Drawing for the job (mm, zero at the part's lowest x, y, z). Coordinates: 2 decimals unless noted, no trailing zeros. Write each loop counter-clockwise with the first axis right and the second up, starting at its lowest first coordinate (ties: lowest second). Pieces come first, ordered by that corner, then holes. Notation, with made-up numbers: (-10.75, -23.75) -> (13.25, -23.75) arc R20 ccw to (13.25, 5.25) -> close; hole circle Ø5 at (15.5, 78.25). An arc over 180 degrees is marked (long way). Write each question's results on one line, items separated by ' | '. Start each with the question number.
Q1. Saw through at A-A on y = 50. Give the cut face in (x, z).
Q2. Saw through at D-D on x = 2.1. Count the separate pieces of the cut face and the enclosed holes in it, and give its area (3 significant figures).
Q3. Saw through at C-C on y = 32. Give the cut face in (x, z).
Q4. Drop a flat-ended pin along its axis: pin 1 Ø5 at (y, z) = (85.39, 75.72) entering from -X. Give the stop position or say it passes through.
Q5. Drill centre lines: line 1 (Y direction, x = 1.1, z = 50); line 2 (Y direction, x = 0.9, z = 91) (1 decimal); line 3 (Z direction, x = 0.4, y = 73.5) (1 decimal). Where is each one in solid material? Low to high.
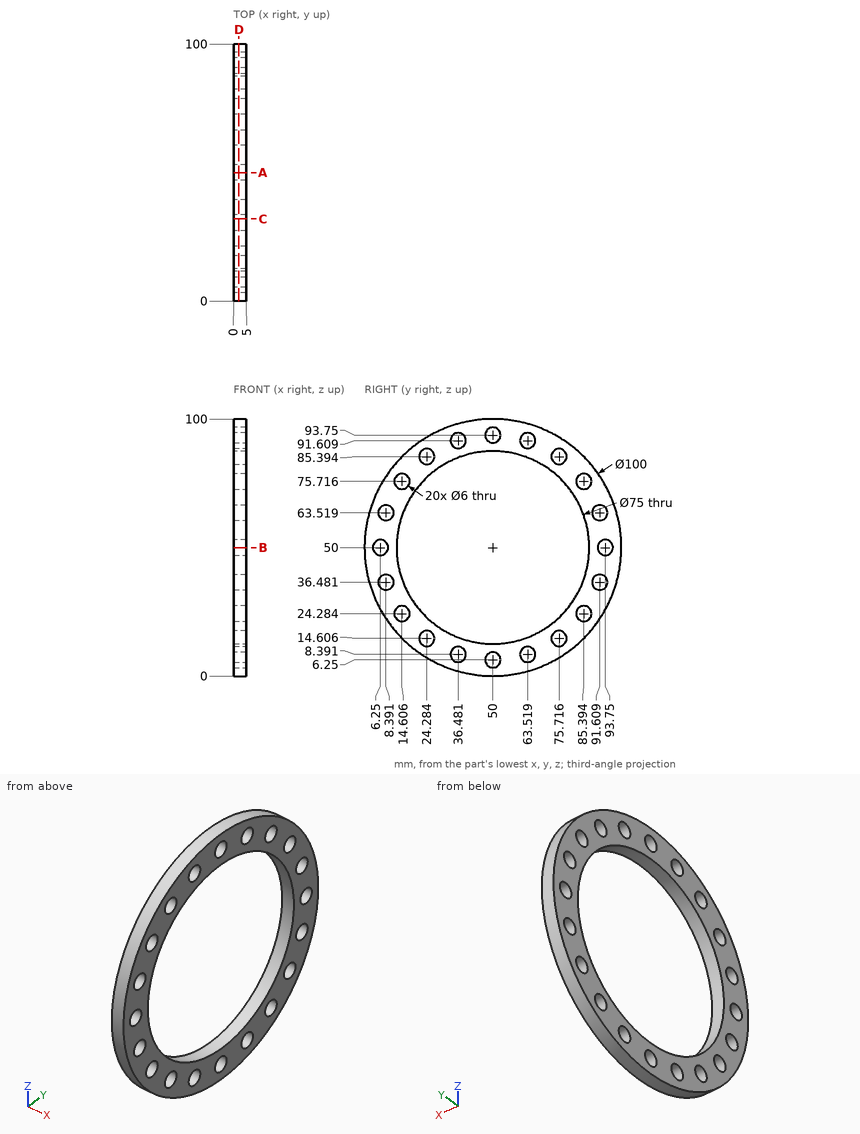
Returned:
1) outline: (0, 0) -> (5, 0) -> (5, 3.25) -> (0, 3.25) -> close; (0, 9.25) -> (5, 9.25) -> (5, 12.5) -> (0, 12.5) -> close; (0, 87.5) -> (5, 87.5) -> (5, 90.75) -> (0, 90.75) -> close; (0, 96.75) -> (5, 96.75) -> (5, 100) -> (0, 100) -> close
2) separate pieces: 1 | enclosed holes: 21 | area: 2,870 mm2
3) outline: (0, 3.35) -> (5, 3.35) -> (5, 17.1) -> (0, 17.1) -> close; (0, 82.9) -> (5, 82.9) -> (5, 96.65) -> (0, 96.65) -> close
4) pin 1: passes through
5) line 1: y = 0 to 3.25, 9.25 to 12.5, 87.5 to 90.75, 96.75 to 100 | line 2: y = 21.4 to 33.5, 39.4 to 48.8, 51.2 to 60.6, 66.5 to 78.6 | line 3: z = 5.9 to 12.6, 16.6 to 20.8, 79.2 to 83.4, 87.4 to 94.1
